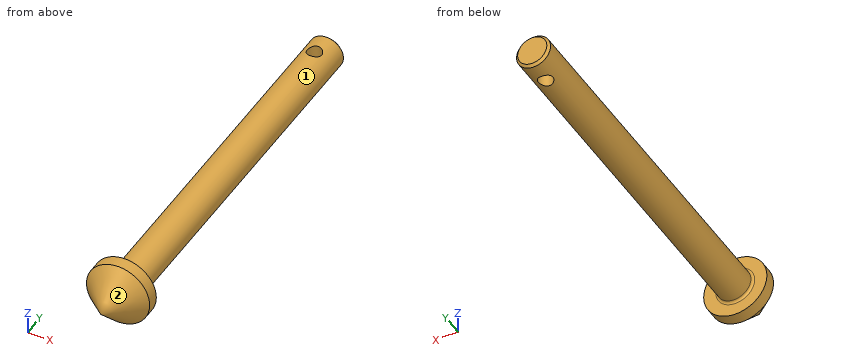
```python
from build123d import *

# Parameters (mm, degrees)
SZKIC2_R                        = 1.5
WYTNIJ_WYCI_GNI_CIE1_DEPTH      = 7.5
WYTNIJ_WYCI_GNI_CIE1_DEPTH_BACK = 7.5
SFAZOWANIE4_SIZE                = 0.5


with BuildPart() as part:
    # Szkic1 → Obrót2 (revolve)
    with BuildSketch(Plane.XY):
        with BuildLine():
            Line((0, 0), (6.5, 6.5))
            Line((6.5, 6.5), (6.5, 9))
            Line((6.5, 9), (4, 9))
            ThreePointArc((4, 9), (3.646446609, 9.146446609), (3.5, 9.5))
            Line((3.5, 9.5), (3.5, 85))
            Line((3.5, 85), (0, 85))
            Line((0, 85), (0, 0))
        make_face()
    revolve(axis=Axis((0, 0, 0), (0, 1, 0)))

    # Szkic2 → Wytnij-wyciągnięcie1 (cut, two sides)
    with BuildSketch(Plane.XY) as wytnij_wyci_gni_cie1_sk:
        with Locations((0, 80)):
            Circle(SZKIC2_R)
    extrude(amount=WYTNIJ_WYCI_GNI_CIE1_DEPTH, mode=Mode.SUBTRACT)
    extrude(wytnij_wyci_gni_cie1_sk.sketch, amount=-WYTNIJ_WYCI_GNI_CIE1_DEPTH_BACK, mode=Mode.SUBTRACT)

    # Sfazowanie4
    sfazowanie4_edges = [part.edges().sort_by_distance(p)[0] for p in [
        (-3.5, 85, 0),
    ]]
    chamfer(sfazowanie4_edges, length=SFAZOWANIE4_SIZE)


solid = part.part
```
CAD build for the part. Positions are in the model's coordinates, mm. Face numbers are marked on the shaded views. A direction names the side the tool comes from. Give positions to 0.01 mm unless a question says otherwise; leave off trailing zeros. Order: outer loops, then holes, each group sorted by start corner. A loop starts at its lowest first (then second) coordinate and runs counter-clockwise, first axis right, second up.
(1) Drill centre lines: L1, parallel to Y at x = 0, z = -1.5; L2, parallel to Y at x = 0, z = 0; L3, parallel to X at y = 80, z = 2.25. Where is each one in solid material? Low to high.
(2) Saw through at A-A, the plane y = 80. Give the cut face in (x, z).
(3) Tool access for the marked faces 1 and 2: list every direction of +Z, -Z, +X, -X, +Y, -Y with a clear straight run to the whole face (end or side of a thin tool).
(4) Saw through at B-B, the plane y = 67. Give the cut face in (x, z), then the cut area to 3 significant figures.
(5) Flat gauge pins, fed straight in: pin 1 (2 mm diameter, centred on x = -5, y = 57, fed in from +Z) (3 decimals); pin 2 (1 mm diameter, centred on x = -2.5, z = 5, fed in from +Y); pin 3 (3 mm diameter, centred on y = 26.5, z = -0.5, fed in from -X); pin 4 (2 mm diameter, centred on y = 13, z = 3.5, fed in from +X). Where does each tip first touch, or does it go through?
Results found:
1. L1: y = 1.5 to 78.5, 81.5 to 85
1. L2: y = 0 to 78.5, 81.5 to 85
1. L3: x = -2.68 to -1.5, 1.5 to 2.68
2. outline: (-1.5, -3.16) - (-1.5, 3.16) arc R3.5 ccw to start; (1.5, -3.16) arc R3.5 ccw to (1.5, 3.16) - close
3. face 1: +Y
3. face 2: -Y
4. outline: circle Ø7 at (0, 0)
4. area: 38.5 mm2
5. pin 1: passes through
5. pin 2: stops at y = 9
5. pin 3: stops at x = -3.5
5. pin 4: stops at x = 2.45
